Could you check a few things on this model? Use its own coordinates, in mm. A direction names the side the tool comes from. Give positions to 0.01 mm unless a question says otherwise; leave off trailing zeros. Loops run counter-clockwise (first coordinate to the right, second up) from the corner with the lowest first, then second, coordinate; pieces in that order, holes last. Notation, with made-up numbers: M 10.25,-31.5 L 51.25,-31.5 A23 cw 51.25,-23.5 Z; hole C -14,25 d7. An arc over 180 degrees is marked long. Answer in a Markdown table with one row per item. Add a question column.
Autodesk Fusion 360 part; units mm, degrees
sketch "Sketch1" plane through (0, 0, 0) normal (0, 0, 1) x (1, 0, 0)
  line L0 (0, 0) -> (-20, 0)
  line L1 (-20, 0) -> (-20, 20)
  line L2 (-20, 20) -> (0, 20)
  line L3 (0, 20) -> (0, 0)
  line L4 (-20, 20) -> (0, 0) construction
  circle A0 centre (-10, 10) radius 2.6
  line L5 (-10, 20) -> (-20, 10)
  line L6 (-20, 10) -> (-34.1421, -4.1421)
  line L7 (-20, 10) -> (-0.3454, 10) construction
  line L8 (-34.1421, -4.1421) -> (-36.2635, -2.0208)
  line L9 (-34.1421, -4.1421) -> (-30.4876, -4.1421) construction
  line L10 (-36.2635, -2.0208) -> (-7.9792, 26.2635)
  line L11 (-36.2635, -2.0208) -> (3.0294, -2.0208) construction
  line L12 (-10, 20) -> (-12.1213, 22.1213)
  line L13 (-20, 0) -> (-34.2426, 0)
  dimension "d5" = 20
  dimension "d6" = 20
  dimension "d7" = 5.2
  dimension "d8" = 135
  dimension "d9" = 20
  dimension "d10" = 135
  dimension "d11" = 3
  dimension "d14" = 45
  dimension "d15" = 40
extrude "Extrude1" add sketch "Sketch1" against normal blind 3 contours L0 L1 L2 L3 L5 | L1 L6 L13 makes body 1
extrude "Extrude2" add sketch "Sketch1" against normal blind 60 separate body contours L1 L6 L10 L13 | L1 L2 L5 L10 makes body 2
sketch "Sketch2" plane through (-17.1213, 17.1213, 0) normal (-0.7071, 0.7071, 0) x (-0.7071, -0.7071, 0)
  line L0 (24.2132, 0) -> (-4.0711, 0)
  line L1 (-4.0711, 0) -> (-4.0711, -60)
  line L2 (-4.0711, -60) -> (24.2132, -60)
  line L3 (24.2132, -60) -> (24.2132, 0)
  line L4 (24.2132, -30) -> (-4.0711, -30) construction
  line L5 (17.1608, -55) -> (20.5608, -55) construction
  line L6 (20.5608, -55) -> (20.5608, -5)
  line L7 (20.5608, -5) -> (17.1608, -5) construction
  line L8 (17.1608, -5) -> (17.1608, -55)
  line L9 (17.1608, -55) -> (20.5608, -5) construction
  line L10 (20.5608, -55) -> (17.1608, -5) construction
  arc A0 (17.1765, -54.7699) -> (20.5452, -54.7699) centre (18.8608, -55) ccw
  arc A1 (20.5452, -5.2301) -> (17.1765, -5.2301) centre (18.8608, -5) ccw
  arc A2 (11.1765, -54.7699) -> (14.5452, -54.7699) centre (12.8608, -55) ccw
  line L11 (14.5608, -55) -> (14.5608, -5)
  line L12 (11.1608, -5) -> (11.1608, -55)
  arc A3 (14.5452, -5.2301) -> (11.1765, -5.2301) centre (12.8608, -5) ccw
  arc A4 (5.1765, -54.7699) -> (8.5452, -54.7699) centre (6.8608, -55) ccw
  line L13 (8.5608, -55) -> (8.5608, -5)
  line L14 (5.1608, -5) -> (5.1608, -55)
  arc A5 (8.5452, -5.2301) -> (5.1765, -5.2301) centre (6.8608, -5) ccw
  arc A6 (-0.8235, -54.7699) -> (2.5452, -54.7699) centre (0.8608, -55) ccw
  line L15 (2.5608, -55) -> (2.5608, -5)
  line L16 (-0.8392, -5) -> (-0.8392, -55)
  arc A7 (2.5452, -5.2301) -> (-0.8235, -5.2301) centre (0.8608, -5) ccw
  point P0 (18.8608, -30)
  dimension "d23" = 3.4
  dimension "d24" = 50
  dimension "d27" = -6
  dimension "d28" = 0
extrude "Extrude3" cut sketch "Sketch2" against normal blind 3 contours L6 L8 A0 A1 | A2 L11 L12 A3 | A4 L13 L14 A5 | A6 L15 L16 A7 bodies 2
combine "Combine1" operation add target body 1 tool bodies 2
equation "holder_depth = 20 mm"
equation "holder_width = 20 mm"
equation "d5 = holder_width"
equation "d6 = holder_depth"
equation "d7 = m5_hole"
equation "d11 = holder_base_height"
equation "holder_base_height = 3 mm"
equation "holder_height = 60 mm"
equation "d23 = m3_hole"
equation "d24 = holder_height - 10 mm"
equation "m3_hole = 3.4 mm"
equation "m5_hole = 5.2 mm"
Item 1: For P1, Ø2, axis at x = -13.5, z = -19, coming from the -Y side; P2, Ø2, axis at y = 8.5, z = -12, coming from the +X side; P3, Ø1, axis at x = -16.5, y = 5.5, coming from the -Z side, each with a flat end and sliding along its axis, tell me the tip position at first contact or that it passes through.
Item 2: Suppose I cut it at A-A (x = -9). List the corners of the cut face in (y, z) for me, then the cut area to 3 significant figures.
Item 3: For faces 1 (the face through (-30.614, 1.537, -30.35)), 2 (the face through (-8.8, 7.693, -1.479)), 3 (the face through (-12, 8, -3)), 4 (the face through (-25.2, 7, -3.3)), 5 (the face through (-19.7, 12.4, -29.6)), which set-ups out of +Z, -Z, +X, -X, +Y, -Y let a thin tool reach every point of the face, with its end or its side?
Item 4: Suppose I cut it at B-B (z = -9). List the corners of the cut face in (x, y) for me, then the cut area to 3 significant figures.
Item 5: If we mould it in two halves opening along Y, with no side actions, what happens to faces 6 (the face through (-26.37, 5.78, -30.35)), 7 (the face through (-21, 11.2, -3.3)), 8 (the face through (0, 10, -1))? For each: +Y half, -Y half, draft (parallel to the pull), parting line (faces both ways), or undercut.
Item 6: I need wall thicknesses on L1, parallel to Y at x = -10, z = -1; L2, parallel to Z at x = -12, y = 14.25; L3, parallel to X at y = 1, z = -10. Which ranges of each line are inside material? Lowest first, please.
Values found:
| question | item | result |
|---|---|---|
| 1 | P1 | y = 15.59 |
| 1 | P2 | x = -21.05 |
| 1 | P3 | z = -3 |
| 2 | outline | M 0,-3 L 7.6,-3 L 7.6,0 L 0,0 Z; M 12.4,-3 L 20,-3 L 20,0 L 12.4,0 Z |
| 2 | area | 45.6 mm² |
| 3 | face 1 | +X, +Y |
| 3 | face 2 | +Z, -Z |
| 3 | face 3 | -Z, +X, -Y |
| 3 | face 4 | none |
| 3 | face 5 | -X, -Y |
| 4 | outline | M -34.24,0 L -30,0 L -29.54,0.46 L -31.66,2.58 Z; M -29.26,4.99 L -27.13,2.87 L -25.3,4.7 L -27.42,6.83 Z; M -25.01,9.23 L -22.89,7.11 L -21.05,8.95 L -23.17,11.07 Z; M -20.77,13.47 L -18.65,11.35 L -16.81,13.19 L -18.93,15.31 Z; M -16.53,17.71 L -14.41,15.59 L -10,20 L -14.24,20 Z |
| 4 | area | 44.1 mm² |
| 5 | face 6 | +Y half |
| 5 | face 7 | undercut |
| 5 | face 8 | draft |
| 6 | L1 | 0 to 7.4, 12.6 to 20 |
| 6 | L2 | -3 to 0 |
| 6 | L3 | -33.24 to -30.08 |
